The listing builds one solid part. Answer for the finished solid, in the listing's coordinates (mm). A direction names the side the tool comes from. Round coordinates to 2 decimals unless told otherwise and drop trailing zeros. Loops run counter-clockwise (first coordinate to the right, second up) from the corner with the lowest first, then second, coordinate; pieces in that order, holes last. Notation, with made-up numbers: M 30,-15 L 60,-15 A37 ccw 60,21 Z; hole C 56.5,-32 d2. An arc over 180 degrees is marked long. Answer as a JSON object with one key per item and string values.
```python
from build123d import *

# Parameters (mm, degrees)
SKETCH1_R                   = 89.825
SKETCH1_R_2                 = 47.825
BOSS_EXTRUDE1_DEPTH         = 10
SKETCH3_R                   = 47.825
TBH_IDK_DEPTH               = 5
EXTRUSION_START             = 5
SKETCH4_R                   = 47.825
EXTRUSION_TO_FUEL_MAN_DEPTH = 5
OX_DOWNCOMER_REACH          = 129.914
OX_PROFILE_R                = 0.914623685


with BuildPart() as part:
    # Sketch1 → Boss-Extrude1 (new body)
    with BuildSketch(Plane(origin=(0, 0, 0), x_dir=(0, 0, -1), z_dir=(1, 0, 0))):
        Circle(SKETCH1_R)
        Circle(SKETCH1_R_2, mode=Mode.SUBTRACT)
    extrude(amount=BOSS_EXTRUDE1_DEPTH)

    # Sketch3 → tbh idk (add)
    with BuildSketch(Plane.ZY):
        Circle(SKETCH3_R)
    extrude(amount=-TBH_IDK_DEPTH)

    # Sketch4 → Extrusion to Fuel Man (add)
    with BuildSketch(Plane.ZY.offset(EXTRUSION_START)):
        Circle(SKETCH4_R)
    extrude(amount=-EXTRUSION_TO_FUEL_MAN_DEPTH)

    # Ox Profile → Ox Downcomer (cut, up to next)
    with BuildSketch(Plane.ZY.offset(5), mode=Mode.PRIVATE) as ox_downcomer_sk1:
        with Locations((0, 23.192029736)):
            Circle(OX_PROFILE_R)
    ox_downcomer_tool1 = extrude(ox_downcomer_sk1.sketch, amount=-OX_DOWNCOMER_REACH, mode=Mode.PRIVATE) & part.part
    # Ox Profile → Ox Downcomer (cut, up to next)
    with BuildSketch(Plane.ZY.offset(5), mode=Mode.PRIVATE) as ox_downcomer_sk2:
        with Locations((0, 35.373170264)):
            Circle(OX_PROFILE_R)
    ox_downcomer_tool2 = extrude(ox_downcomer_sk2.sketch, amount=-OX_DOWNCOMER_REACH, mode=Mode.PRIVATE) & part.part
    add(ox_downcomer_tool1.solids().sort_by_distance((-5, 23.19203, 0))[0], mode=Mode.SUBTRACT)
    add(ox_downcomer_tool2.solids().sort_by_distance((-5, 35.37317, 0))[0], mode=Mode.SUBTRACT)


solid = part.part
```
Item 1: Determine the mould class of faces 1 (the face through (-2.535, 14.365, 45.617)), 2 (the face through (-5, 1, -1)), 3 (the face through (7.465, 14.365, -45.617)) for opening direction Y: released by +Y, released by -Y, zero draft, split by the parting line, or undercut.
Values follow:
{"face 1": "split by the parting line", "face 2": "zero draft", "face 3": "undercut"}
Item 2: Straight lines are drawn through the part: line 1 (Y direction, x = -1.25, z = 0) (3 decimals); line 2 (Y direction, x = 1, z = 0) (3 decimals); line 3 (X direction, y = -49, z = 34). For each, find the intervals that lie inside material, in ascending order.
Values follow:
{"line 1": "-47.825 to 22.277, 24.107 to 34.459, 36.288 to 47.825", "line 2": "-89.825 to 22.277, 24.107 to 34.459, 36.288 to 89.825", "line 3": "0 to 10"}
Item 3: The part is cut by section B-B (z = -22.5). Give the vertices of the cut face in (x, y), then the cut area to 3 significant figures.
Values follow:
{"outline": "M -5,-42.2 L 0,-42.2 L 0,-86.96 L 10,-86.96 L 10,-42.2 L 5,-42.2 L 5,42.2 L 10,42.2 L 10,86.96 L 0,86.96 L 0,42.2 L -5,42.2 Z", "area": "1,740 mm^2"}
Item 4: Which of the six approach directions +Z, -Z, +X, -X, +Y, -Y give full straight-line access (tool end or side, diameter ignored) to faces 4 (the face through (5, 1, -1)), 5 (the face through (0, -39, 39)), 6 (the face through (4.93, -87.69, 19.47))?
Values follow:
{"face 4": "+X", "face 5": "-X", "face 6": "+X, -X"}
Item 5: Flat-ended cylindrical pins translate along their axes: P1, Ø12, axis at y = -54.5, z = -59.5, coming from the -X side; P2, Ø1, axis at x = -2.5, z = -4.5, coming from the +Y side; P3, Ø5, axis at x = 6.5, y = -62.5, coming from the -Z side; P4, Ø1.5, axis at y = 23.19, z = 0, coming from the -X side. Find the tip coordinate at first contact, or state that the pin passes through.
Values follow:
{"P1": "x = 0", "P2": "y = 47.66", "P3": "z = -66.85", "P4": "through"}
Item 6: The part is cut by section C-C (x = 7.75). Give the vertices of the cut face in (y, z) (3 decimals), then the cut area to 3 significant figures.
Values follow:
{"outline": "C 0,0 d179.65; hole C 0,0 d95.65", "area": "18,200 mm^2"}
Item 7: The part is cut by section D-D (y = 60.5). Give the vertices of the cut face in (x, z).
Values follow:
{"outline": "M 0,-66.39 L 10,-66.39 L 10,66.39 L 0,66.39 Z"}
Item 8: The part is cut by section A-A (y = 0). Give the vertices of the cut face in (x, z) (3 decimals).
Values follow:
{"outline": "M -5,-47.825 L 0,-47.825 L 0,-89.825 L 10,-89.825 L 10,-47.825 L 5,-47.825 L 5,47.825 L 10,47.825 L 10,89.825 L 0,89.825 L 0,47.825 L -5,47.825 Z"}
